Autodesk Inventor part; units mm, degrees
ref_plane "YZ Plane" through (0, 0, 0) normal (1, 0, 0) x (0, 1, 0)
ref_plane "XZ Plane" through (0, 0, 0) normal (0, 1, 0) x (-1, 0, 0)
ref_plane "XY Plane" through (0, 0, 0) normal (0, 0, 1) x (1, 0, 0)
sketch "Skizze1" plane through (0, 0, 0) normal (0, 0, 1) x (1, 0, 0)
  line L0 (-6, 12) -> (48, 12)
  line L1 (48, 12) -> (48, -12)
  line L2 (48, -12) -> (-6, -12)
  line L3 (-16.8, 0) -> (58.8, 0)
  line L4 (0, 16.8) -> (0, -16.8)
  line L5 (-6, 12) -> (-6, -12)
  point P0 (0, 0)
  dimension "d2" = 24
  dimension "d3" = 54
  dimension "d59" = 6
extrude "Extrusion1" add sketch "Skizze1" along normal blind 6
sketch "Skizze2" plane through (0, 0, 0) normal (0, 0, -1) x (-1, 0, 0)
  line L0 (-48, -12) -> (6, -12)
  line L1 (-48, 12) -> (-48, -12)
  line L2 (-48, 12) -> (6, 12)
  line L3 (6, -12) -> (-48, -12)
  line L4 (-48, -12) -> (-48, 12)
  line L5 (-48, 12) -> (6, 12)
  line L6 (6, 12) -> (6, -12)
  point P0 (0, 0)
extrude "Extrusion2" cut sketch "Skizze2" against normal blind 2
sketch "Skizze3" plane through (0, 0, 2) normal (0, 0, -1) x (-1, 0, 0)
  line L0 (6, -12) -> (-48, -12)
  line L1 (-48, -12) -> (-48, 12)
  line L2 (-48, 12) -> (6, 12)
  line L3 (-48, -12) -> (-44, -12)
  line L4 (-44, -12) -> (-44, 12)
  line L5 (-44, 12) -> (-48, 12)
  line L6 (-48, 12) -> (-48, -12)
  point P0 (0, 0)
  point P1 (0, -12.5)
  dimension "d9" = 4
extrude "Extrusion3" cut sketch "Skizze3" against normal blind 2
sketch "Skizze4" plane through (0, 0, 6) normal (0, 0, 1) x (1, 0, 0)
  line L0 (48, -12) -> (48, 12)
  line L1 (-17, 0) -> (60, 0)
  point P0 (0, 0)
  point P1 (46, 0)
  dimension "d12" = 2
hole "Bohrung1" at (46, 0, 6) direction (0, 0, -1) diameter 2 end through all
pattern_linear "Rechteckige Anordnung1" count 5 spacing 5 along (0, 1, 0) of "Bohrung1" first direction both ways yes
sketch "Skizze7" plane through (0, 0, 2) normal (0, 0, -1) x (-1, 0, 0)
  line L0 (-44, 12) -> (-44, -12)
  line L1 (6, -12) -> (-44, -12)
  line L2 (6, 12) -> (6, -12)
  line L3 (-44, 12) -> (6, 12)
  line L4 (-48, 12) -> (6, 12)
  line L5 (6, -12) -> (0, -12)
  line L6 (0, -12) -> (0, 12)
  line L7 (0, 12) -> (6, 12)
  line L8 (6, 12) -> (6, -12)
  point P0 (0, 0)
extrude "Extrusion4" add sketch "Skizze7" along normal blind 2.8 contours L3 L2 L1 L6
sketch "Skizze8" plane through (0, 0, -0.8) normal (0, 0, -1) x (-1, 0, 0)
  line L0 (6, -12) -> (6, 12)
  line L1 (6, 12) -> (0, 12)
  line L2 (0, 12) -> (0, -12)
  line L3 (0, -12) -> (6, -12)
  line L4 (-58.8, 0) -> (16.8, 0)
  line L5 (6, 12) -> (0, 12)
  line L6 (0, 12) -> (0, 24)
  line L7 (0, 24) -> (6, 24)
  line L8 (6, 24) -> (6, 12)
  line L9 (6, -12) -> (-48, -12)
  line L10 (6, -12) -> (0, -12)
  line L11 (0, -12) -> (0, -24)
  line L12 (0, -24) -> (6, -24)
  line L13 (6, -24) -> (6, -12)
  line L14 (6, -12) -> (6, 12)
  dimension "d67" = 48
extrude "Extrusion5" add sketch "Skizze8" against normal up to surface (6.8 mm away)
sketch "Skizze9" plane through (0, 0, 6) normal (0, 0, 1) x (1, 0, 0)
  line L0 (0, -12) -> (48, -12)
  line L1 (48, -12) -> (48, 12)
  line L2 (48, 12) -> (0, 12)
  line L3 (0, 24) -> (0, 12)
  line L4 (-6, 24) -> (0, 24)
  line L5 (-6, -24) -> (-6, 24)
  line L6 (0, -24) -> (-6, -24)
  line L7 (0, -12) -> (0, -24)
  circle A0 centre (46, 0) radius 1
  circle A1 centre (46, -10) radius 1
  circle A2 centre (46, -5) radius 1
  circle A3 centre (46, 5) radius 1
  circle A4 centre (46, 10) radius 1
  line L8 (44, 12) -> (0, 12)
  arc A5 (0, 12) -> (3.6, 12) centre (1.8, 12) ccw
  line L9 (0, -12) -> (44, -12)
  arc A6 (3.6, -12) -> (0, -12) centre (1.8, -12) ccw
  line L10 (-17, 0) -> (60, 0)
  point P0 (0, 0)
  dimension "d68" = 1.8
extrude "Extrusion6" cut sketch "Skizze9" against normal through all contours A6 L0 | L2 A5
fillet "Rundung1" radius 2 4 edges at (0, -12, 4) (3.6, -12, 4) (0, 12, 4) (3.6, 12, 4)
sketch "Skizze10" plane through (0, 0, -0.8) normal (0, 0, -1) x (-1, 0, 0)
  line L0 (0, -24) -> (0, 24)
  line L1 (-58.8, 0) -> (16.8, 0)
  line L2 (0, -22) -> (6, -22) construction
  line L3 (6, 24) -> (6, -24)
  point P0 (0, 0)
  point P1 (3, -22)
  point P2 (3, 22)
  dimension "d72" = 22
hole "Bohrung4" at (-3, -22, -0.8) at (-3, 22, -0.8) direction (0, 0, 1) diameter 1.567 end through all
fillet "Rundung2" radius 1 4 edges at (0, 24, 2.6) (-6, 24, 2.6) (0, -24, 2.6) (-6, -24, 2.6)
sketch "Skizze11" plane through (0, 0, -0.8) normal (0, 0, -1) x (-1, 0, 0)
  arc A0 (5, -24) -> (6, -23) centre (5, -23) ccw
  line L0 (6, 23) -> (6, -23)
  arc A1 (6, 23) -> (5, 24) centre (5, 23) ccw
  line L1 (1, 24) -> (5, 24)
  arc A2 (1, 24) -> (0, 23) centre (1, 23) ccw
  line L2 (0, -23) -> (0, 23)
  arc A3 (0, -23) -> (1, -24) centre (1, -23) ccw
  line L3 (5, -24) -> (1, -24)
  circle A4 centre (3, -22) radius 0.7835
  circle A5 centre (3, 22) radius 0.7835
  point P0 (0, 0)
extrude "Extrusion7" cut sketch "Skizze11" against normal blind 0.2
properties part number "Kicker Chip" material "Aluminium 6061"
The model under review builds one solid part; all positions refer to its coordinate system, in mm. A direction names the side the tool comes from. Round coordinates to 2 decimals unless told otherwise and drop trailing zeros. Loops run counter-clockwise (first coordinate to the right, second up) from the corner with the lowest first, then second, coordinate; pieces in that order, holes last. Notation, with made-up numbers: (74, 79.25) -> (96, 79.25) arc R17 ccw to (96, 89.25) -> close; hole circle Ø11 at (-3.5, 73.5). An arc over 180 degrees is marked (long way). Answer as CSV lines item,"result".
1) To check wall thickness, follow line 1 along Y through (x, z) = (46, 4.55); line 2 along X through (y, z) = (22, 3.5); line 3 along Y through (x, z) = (-3, 1.5). State the ranges of each line that lie inside material, in increasing order. Write a range as from..to.
Geometry results:
line 1,"y = -12..-11, -9..-6, -4..-1, 1..4, 6..9, 11..12"
line 2,"x = -6..-3.78, -2.22..0"
line 3,"y = -24..-22.78, -21.22..21.22, 22.78..24"
2) Tool access review of faces 1 (the face through (0, 0, 1)), 2 (the face through (47.4, 0.2, 4)), 3 (the face through (4.045, 11.74, 3.972)), 4 (the face through (26, -12, 4)), 5 (the face through (4.07, -11.754, 3.972)): name each direction out of +Z, -Z, +X, -X, +Y, -Y from which nothing blocks a thin tool from reaching the whole face with its end or side.
Geometry results:
face 1,"-Z, +X"
face 2,"-Z, +X, +Y, -Y"
face 3,"+Z, -Z, +Y"
face 4,"+Z, -Z, +X, -Y"
face 5,"+Z, -Z, -Y"
3) For P1, Ø4, axis at x = 10, y = 10, coming from the -Z side; P2, Ø2.5, axis at x = 46, y = -5, coming from the +Z side; P3, Ø3, axis at x = 46, y = -10, coming from the -Z side; P4, Ø3.5, axis at y = 0.5, z = 1, coming from the +X side, all flat-tipped, find the tip position at first contact; note any pin that passes through.
Geometry results:
P1,"stops at z = 2"
P2,"stops at z = 6"
P3,"stops at z = 4"
P4,"stops at x = 44"
4) Add section C-C on z = 2.75. Write out the cut boundary in (x, y), plus the area to 3 significant figures.
Geometry results:
outline,"(-6, -23) arc R1 ccw to (-5, -24) -> (-1, -24) arc R1 ccw to (0, -23) -> (0, -12) arc R1.8 cw to (3.33, -11.05) arc R2 ccw to (5.03, -12) -> (44, -12) -> (44, 12) -> (5.03, 12) arc R2 ccw to (3.33, 11.05) arc R1.8 cw to (0, 12) -> (0, 23) arc R1 ccw to (-1, 24) -> (-5, 24) arc R1 ccw to (-6, 23) -> close; hole circle Ø1.57 at (-3, -22); hole circle Ø1.57 at (-3, 22)"
area,"1,330 mm²"
5) Add section B-B on x = 46. Write out the cut boundary in (y, z), plus the area to 3 significant figures.
Geometry results:
outline,"(-12, 4) -> (-11, 4) -> (-11, 6) -> (-12, 6) -> close; (-9, 4) -> (-6, 4) -> (-6, 6) -> (-9, 6) -> close; (-4, 4) -> (-1, 4) -> (-1, 6) -> (-4, 6) -> close; (1, 4) -> (4, 4) -> (4, 6) -> (1, 6) -> close; (6, 4) -> (9, 4) -> (9, 6) -> (6, 6) -> close; (11, 4) -> (12, 4) -> (12, 6) -> (11, 6) -> close"
area,"28.0 mm²"
6) Add section D-D on y = 22. Write out the cut boundary in (x, z).
Geometry results:
outline,"(-6, -0.6) -> (-3.78, -0.6) -> (-3.78, 6) -> (-6, 6) -> close; (-2.22, -0.6) -> (0, -0.6) -> (0, 6) -> (-2.22, 6) -> close"
7) Draft analysis for pull direction X (two halves, no side actions). For faces 6 (the face through (-6, 0, 3)), 7 (the face through (44, 0, 3)), 8 (the face through (27, 12, 4)), 9 (the face through (45, -5, 5)), state which applies: pulls with the +X half, pulls with the -X half, needs draft (parallel to the pull), parting line crosses it, or undercut.
Geometry results:
face 6,"pulls with the -X half"
face 7,"pulls with the +X half"
face 8,"needs draft"
face 9,"undercut"
8) Add section A-A on y = 0. Write out the cut boundary in (x, z).
Geometry results:
outline,"(-6, -0.6) -> (0, -0.6) -> (0, 2) -> (44, 2) -> (44, 4) -> (45, 4) -> (45, 6) -> (-6, 6) -> close; (47, 4) -> (48, 4) -> (48, 6) -> (47, 6) -> close"
